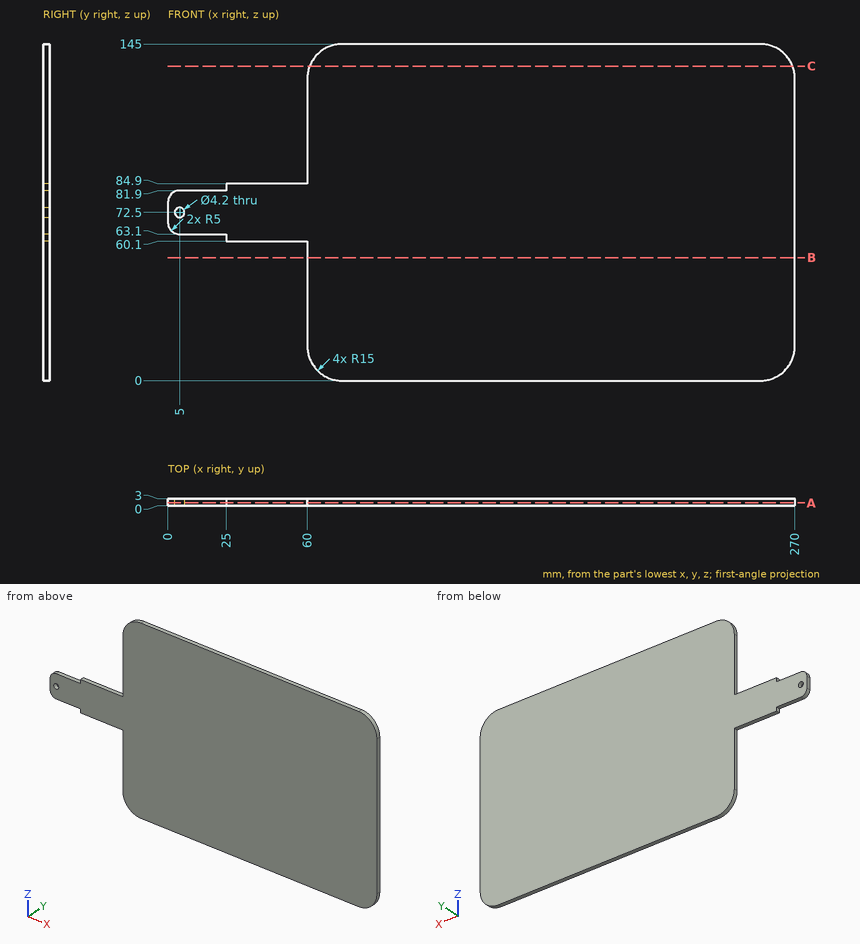
Can you work these out from the drawing? Everything is in mm from the part's minimum corner. Give positions to 0.01 mm unless a question says otherwise; leave off trailing zeros. Loops run counter-clockwise (first coordinate to the right, second up) from the corner with the lowest first, then second, coordinate; pieces in that order, holes last. Notation, with made-up numbers: M 45,-20 L 57,-20 A15 cw 57,-15 Z; hole C 50.25,-15 d2. An arc over 180 degrees is marked long. Put each result on its own line as item: value. Start each with the question number.
(1) I want a section at C-C on z = 135.5. Please give me the cut outline in (x, y), then the cut area to 3 significant figures.
(2) I need wall thicknesses on line 1 along X through (y, z) = (1.95, 34.5); line 2 along X through (y, z) = (2.25, 81). Which ranges of each line are inside material? Lowest first, please. Write a range as [from, to].
(3) I want a section at A-A on y = 1.2. Please give me the cut outline in (x, z).
(4) I want a section at B-B on z = 53. Please give me the cut outline in (x, y).
(5) Will these pins go through, and if not, where does the flat tip stop? pin 1 Ø1.5 at (x, y) = (12, 2) entering from +Z; pin 2 Ø1.5 at (x, y) = (19, 1) entering from -Z; pin 3 Ø1.5 at (x, y) = (41, 1) entering from -Z.
Answer block:
1. outline: M 61.04,0 L 268.96,0 L 268.96,3 L 61.04,3 Z
1. area: 624 mm^2
2. line 1: [60, 270]
2. line 2: [2.14, 270]
3. outline: M 0,68.1 A5 ccw 5,63.1 L 25,63.1 L 25,60.1 L 60,60.1 L 60,15 A15 ccw 75,0 L 255,0 A15 ccw 270,15 L 270,130 A15 ccw 255,145 L 75,145 A15 ccw 60,130 L 60,84.9 L 25,84.9 L 25,81.9 L 5,81.9 A5 ccw 0,76.9 Z; hole C 5,72.5 d4.2
4. outline: M 60,0 L 270,0 L 270,3 L 60,3 Z
5. pin 1: z = 81.9
5. pin 2: z = 63.1
5. pin 3: z = 60.1
